Build history of the part. All positions in model axes, mm. Face numbers are marked on the shaded views. A direction names the side the tool comes from. Round coordinates to 2 decimals unless told otherwise and drop trailing zeros. Write each loop counter-clockwise with the first axis right and the second up, starting at its lowest first coordinate (ties: lowest second). Pieces come first, ordered by that corner, then holes.
from build123d import *

# Parameters (mm, degrees)
SKETCH1_W                    = 44.45
SKETCH1_H                    = 88.9
BASE_FLANGE1_DEPTH           = 3.175
EDGE_FLANGE1_STRIP_W         = 19.05
EDGE_FLANGE1_STRIP_H         = 3.175
EDGE_FLANGE1_STRIP_CUT_DEPTH = 88.9
EDGE_FLANGE1_DEPTH           = 88.9
BOSS_EXTRUDE1_DEPTH          = 3.175
F_1_4_START                  = -3.175
F_1_4_CLEARANCE_SLOT1_DEPTH  = 3.175
F_1_4_CLEARANCE_HOLE1_D      = 6.7564
CUT_EXTRUDE1_DEPTH           = 139.903982124
FILLET1_R                    = 12.7
FILLET2_R                    = 6.35


# Read off the part's stored shape, not the designer's step: 1/4 Clearance Slot1
# Sheet-metal steps are written as plain solids
with BuildPart() as part:
    # Sketch1 → Base-Flange1 (new body)
    with BuildSketch(Plane.XY):
        with Locations((-22.225, 44.45)):
            Rectangle(SKETCH1_W, SKETCH1_H)
    extrude(amount=-BASE_FLANGE1_DEPTH)

    # Edge-Flange1 strip (across the edge) → Edge-Flange1 strip cut (cut)
    with BuildSketch(Plane(origin=(0, 0, 0), x_dir=(-1, 0, 0), z_dir=(0, 1, 0))):
        with Locations((-3.175, -1.5875)):
            Rectangle(EDGE_FLANGE1_STRIP_W, EDGE_FLANGE1_STRIP_H)
    extrude(amount=EDGE_FLANGE1_STRIP_CUT_DEPTH, mode=Mode.SUBTRACT)

    # Edge-Flange1 section (across the edge) → Edge-Flange1 (add)
    with BuildSketch(Plane(origin=(0, 0, 0), x_dir=(-1, 0, 0), z_dir=(0, 1, 0))):
        with BuildLine():
            Line((0, 3.175), (0, 14.2875))
            Line((0, 14.2875), (3.175, 14.2875))
            Line((3.175, 14.2875), (3.175, 3.175))
            ThreePointArc((3.175, 3.175), (4.10493597, 0.92993597), (6.35, 0))
            Line((6.35, 0), (6.35, -3.175))
            ThreePointArc((6.35, -3.175), (1.859871939, -1.315128061), (0, 3.175))
        make_face()
    extrude(amount=EDGE_FLANGE1_DEPTH)

    # Sketch9 → Boss-Extrude1 (add)
    with BuildSketch(Plane.ZY.offset(3.175)):
        Polygon((35.543004115, -1.859615648), (92.475531111, -6.840566346), (98.425, 61.162174233), (41.492473004, 66.143124931), (14.2875, 88.9), (14.2875, 0), align=None)
    extrude(amount=-BOSS_EXTRUDE1_DEPTH)

    # 1/4 Clearance Slot1 outline → 1/4 Clearance Slot1 (cut)
    with BuildSketch(Plane.XY.offset(F_1_4_START)):
        with BuildLine():
            Line((-31.5468, 12.4968), (-25.6032, 12.4968))
            ThreePointArc((-25.6032, 12.4968), (-22.225, 15.875), (-25.6032, 19.2532))
            Line((-25.6032, 19.2532), (-31.5468, 19.2532))
            ThreePointArc((-31.5468, 19.2532), (-34.925, 15.875), (-31.5468, 12.4968))
        make_face()
        with BuildLine():
            Line((-31.5468, 66.4718), (-25.6032, 66.4718))
            ThreePointArc((-25.6032, 66.4718), (-22.225, 69.85), (-25.6032, 73.2282))
            Line((-25.6032, 73.2282), (-31.5468, 73.2282))
            ThreePointArc((-31.5468, 73.2282), (-34.925, 69.85), (-31.5468, 66.4718))
        make_face()
    extrude(amount=F_1_4_CLEARANCE_SLOT1_DEPTH, mode=Mode.SUBTRACT)

    # 1/4 Clearance Hole1 (through all)
    with Locations(Plane.ZY.offset(3.175)):
        with Locations((68.851858569, 51.000976916), (49.301554713, 9.685179085), (80.930736378, 6.917984253)):
            Hole(F_1_4_CLEARANCE_HOLE1_D / 2)

    # Sketch16 → Cut-Extrude1 (cut, through all)
    with BuildSketch(Plane.ZY.offset(3.175)):
        Polygon((82.610409168, 62.545771649), (78.874696144, 19.846376402), (94.689286976, 18.462778986), (98.425, 61.162174233), align=None)
    extrude(amount=-CUT_EXTRUDE1_DEPTH, mode=Mode.SUBTRACT)

    # Fillet1
    # the kernel refuses this fillet: 12.7 mm, written as the material it adds along each edge
    with BuildSketch(Plane(origin=(0, 0, 14.2875), x_dir=(0, 0, -1), z_dir=(-1, 0, 0))) as fillet1_piece_1:
        with BuildLine():
            CenterArc((FILLET1_R * 0.0436609429085, FILLET1_R), FILLET1_R, 265, 5)
            Line((-FILLET1_R * 0.0434947998391, FILLET1_R * 0.00380530190825), (0, 0))
            Line((0, 0), (FILLET1_R * 0.0436609429085, 0))
        make_face()
    extrude(amount=3.175)
    with BuildSketch(Plane(origin=(-3.175, 66.143124931, 41.492473004), x_dir=(-2.6754118461414173e-15, 0.6416153350460713, -0.7670265717911718), z_dir=(1, 0, 0))) as fillet1_piece_2:
        with BuildLine():
            CenterArc((FILLET1_R * 0.314458316587, FILLET1_R), FILLET1_R, 235.087623307, 34.912376693)
            Line((-FILLET1_R * 0.257864707828, FILLET1_R * 0.179971734802), (0, 0))
            Line((0, 0), (FILLET1_R * 0.314458316587, 0))
        make_face()
    extrude(amount=3.175)
    # the kernel refuses this fillet: 12.7 mm, written as the material it takes off along each edge
    with BuildSketch(Plane(origin=(11.528568508, 88.9, 14.2875), x_dir=(0, 0, -1), z_dir=(-1, 0, 0))) as fillet1_2_piece_1:
        with BuildLine():
            CenterArc((FILLET1_R * 0.363104519926, FILLET1_R), FILLET1_R, 230.087623307, 39.912376693)
            Line((-FILLET1_R * 0.27851081512, FILLET1_R * 0.232973428209), (0, 0))
            Line((0, 0), (FILLET1_R * 0.363104519926, 0))
        make_face()
    extrude(amount=26.232137015, mode=Mode.SUBTRACT)

    # Fillet2
    fillet2_edges = [part.edges().sort_by_distance(p)[0] for p in [
        (-1.5875, 18.462778986, 94.689286976),
        (-1.5875, 62.545771649, 82.610409168),
        (-1.5875, 19.846376402, 78.874696144),
        (-1.5875, -6.840566346, 92.475531111),
        (-44.45, 88.9, -1.5875),
        (-44.45, 0, -1.5875),
    ]]
    fillet(fillet2_edges, radius=FILLET2_R)


solid = part.part
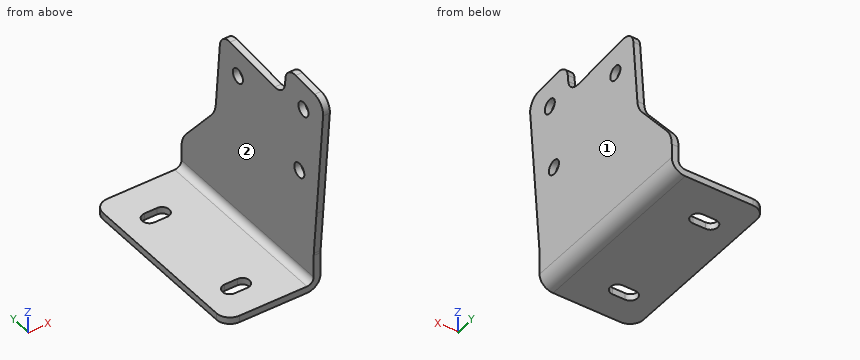
1) Slice it at A-A (z = 67). Write the cut outline in (x, y) (1 decimal).
Results:
outline: (-3.2, -4.6) - (0, -4.6) - (0, 48.2) - (-3.2, 48.2) - close; (-3.2, 53.8) - (0, 53.8) - (0, 63.9) - (-3.2, 63.9) - close
2) Slice it at C-C (x = -16.5). Write the cut outline in (y, z) (3 decimals), plus the area to 3 significant figures.
Results:
outline: (0, -3.175) - (88.9, -3.175) - (88.9, 0) - (0, 0) - close
area: 282 mm2
3) Slice it at B-B (y = 16). Write the cut outline in (x, z) (3 decimals).
Results:
outline: (-44.45, -3.175) - (-34.923, -3.175) - (-34.923, 0) - (-44.45, 0) - close; (-22.227, -3.175) - (-6.35, -3.175) arc R6.35 ccw to (0, 3.175) - (0, 93.229) - (-3.175, 93.229) - (-3.175, 3.175) arc R3.175 cw to (-6.35, 0) - (-22.227, 0) - close
4) Slice it at D-D (y = 43). Write the cut outline in (x, z) (3 decimals), plus the area to 3 significant figures.
Results:
outline: (-44.45, -3.175) - (-6.35, -3.175) arc R6.35 ccw to (0, 3.175) - (0, 80.9) - (-3.175, 80.9) - (-3.175, 3.175) arc R3.175 cw to (-6.35, 0) - (-44.45, 0) - close
area: 391 mm2
5) Pin check, flat tips, straight feed: pin 1 Ø1 at (y, z) = (22.5, 36) entering from +X; pin 2 Ø13.5 at (x, z) = (-19.5, 1.5) entering from -Y; pin 3 Ø6 at (x, y) = (-21, 48.5) entering from +Z; pin 4 Ø8 at (y, z) = (63.5, 33) entering from -X (3 decimals). Stop position of each tip, or through.
Results:
pin 1: stops at x = 0
pin 2: stops at y = 0
pin 3: stops at z = 0
pin 4: stops at x = -3.175
6) Wall check: L1, parallel to X at y = 5, z = 22 (3 decimals); L2, parallel to X at y = 16, z = 2. Give the ranges that are in metal, low to high.
Results:
L1: x = -3.175 to 0
L2: x = -3.4 to -0.11
7) Which spindle directions (+Z, -Z, +X, -X, +Y, -Y) get a long thin tool onto all of the face, cutting with end or side? Do the marked faces 1 and 2. Say none if no direction does.
Results:
face 1: +Z, -Z, +X, +Y, -Y
face 2: +Z, -X, +Y, -Y
